Source: CAD feature listing. Evaluate the final solid. Frame: model axes, mm. Face numbers are marked on the shaded views. A direction names the side the tool comes from. Give positions to 0.01 mm unless a question says otherwise; leave off trailing zeros. Order: outer loops, then holes, each group sorted by start corner. A loop starts at its lowest first (then second) coordinate and runs counter-clockwise, first axis right, second up. Notation, with made-up numbers: M -2.75,-4.75 L 12.25,-4.75 A19 ccw 12.25,13.25 Z; hole C 73.5,84.5 d9. An arc over 180 degrees is marked long. Use CSV: the item, a comma, the result in double quotes. Start each with the question number.
Item 1: Section query B-B on y = 0. Return loops of the section in (x, z), and give its area (3 significant figures).
Item 2: Section query C-C on z = -7. Return loops of the section in (x, y).
Item 3: First-contact query: pin 1 (7 mm diameter, centred on x = -3.5, y = -6.5, fed in from +Z); pin 2 (2 mm diameter, centred on x = 1.5, z = -11.5, fed in from -Y); pin 3 (8 mm diameter, centred on y = 6.5, z = 6.5, fed in from -X); pin 4 (5 mm diameter, centred on y = 7.5, z = -10.5, fed in from +X). Flat tips, straight axial feed; report the tip coordinate or a pass-through.
Item 4: Access query for the marked faces 4 and 5. Directions: +Z, -Z, +X, -X, +Y, -Y. A direction counts if a zero-diameter tool reaches every point of the face in a straight line with its end or side. Return the directions, or none.
Item 5: Pull-direction query (Z, two-part tool) for the marked faces 1, 2 and 3; classes: +Z half, -Z half, draft (parallel to the pull), parting line (faces both ways), or undercut.
Item 6: Section query A-A on y = -7.75. Return loops of the section in (x, z), and give its area (3 significant figures).
Item 7: Ray query, probe 1 along Y at (x, z) = (-9.5, -2); probe 2 along Z at (x, y) = (-4.5, 9); probe 3 along X at (y, z) = (-12.5, -6.5). Return the intervals inside material, ascending. Write a range as from..to.
Item 8: Section query D-D on x = 5. Return loops of the section in (y, z).
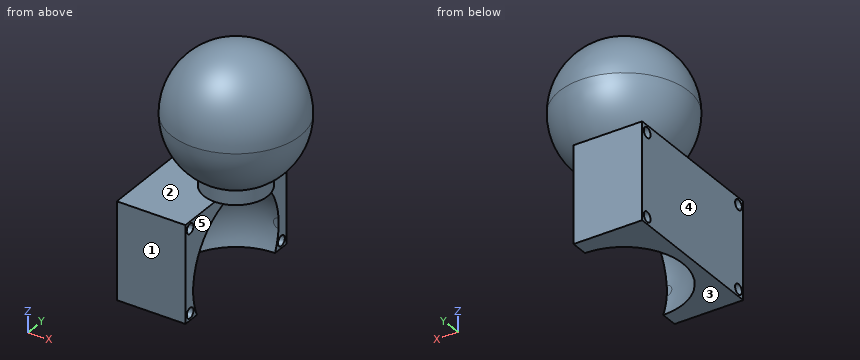
from build123d import *

# Parameters (mm, degrees)
F2_R     = 6.2596868845
F3_DEPTH = 3.048
F4_R     = 1
F5_DEPTH = 13.5


with BuildPart() as f1:
    # F0 (on Right) → F1 (revolve)
    with BuildSketch(Plane.YZ):
        with BuildLine():
            ThreePointArc((0, 1.1509964916), (8.9802561211, 4.8707403706), (12.7, 13.8509964916))
            ThreePointArc((12.7, 13.8509964916), (8.9802561211, 22.8312526127), (0, 26.5509964916))
            Line((0, 26.5509964916), (0, 1.1509964916))
        make_face()
    revolve(axis=Axis((0, 0, 13.8509964916), (0, 0, -1)))

    # F2 (on Top) → F3 (join)
    with BuildSketch(Plane.XY):
        Circle(F2_R)
    extrude(amount=F3_DEPTH)

    # F4 (on Right) → F5 (join)
    with BuildSketch(Plane.YZ):
        with BuildLine():
            Line((-13.603, 0), (-15, 0))
            Line((-15, 0), (-15, -1.397))
            Line((-15, -1.397), (-14.603, -1.397))
            ThreePointArc((-14.603, -1.397), (-14.3101067812, -0.6898932188), (-13.603, -0.397))
            Line((-13.603, -0.397), (-13.603, 0))
        make_face()
        with BuildLine():
            Line((15, 0), (-13.603, 0))
            Line((-13.603, 0), (-13.603, -0.397))
            ThreePointArc((-13.603, -0.397), (-12.8958932188, -0.6898932188), (-12.603, -1.397))
            ThreePointArc((-12.603, -1.397), (-13.603, -2.397), (-14.603, -1.397))
            Line((-14.603, -1.397), (-15, -1.397))
            Line((-15, -1.397), (-15, -12.8640756011))
            Line((-15, -12.8640756011), (-12.6600748075, -12.8640756011))
            ThreePointArc((-12.6600748075, -12.8640756011), (0, -1.170309107), (12.6600748075, -12.8640756011))
            Line((12.6600748075, -12.8640756011), (15, -12.8640756011))
            Line((15, -12.8640756011), (15, 0))
        make_face()
        with Locations((13.5173769371, -1.397)):
            Circle(F4_R, mode=Mode.SUBTRACT)
        with BuildLine():
            Line((-12.6600748075, -12.8640756011), (-15, -12.8640756011))
            Line((-15, -12.8640756011), (-15, -19.05))
            Line((-15, -19.05), (-11.5957234467, -19.05))
            ThreePointArc((-11.5957234467, -19.05), (-12.4208632505, -16.518356711), (-12.7, -13.870309107))
            ThreePointArc((-12.7, -13.870309107), (-12.6900147765, -13.3667964733), (-12.6600748075, -12.8640756011))
        make_face()
        with Locations((-13.603, -17.6556983136)):
            Circle(F4_R, mode=Mode.SUBTRACT)
        with BuildLine():
            Line((15, -19.05), (15, -12.8640756011))
            Line((15, -12.8640756011), (12.6600748075, -12.8640756011))
            ThreePointArc((12.6600748075, -12.8640756011), (12.6900147765, -13.3667964733), (12.7, -13.870309107))
            ThreePointArc((12.7, -13.870309107), (12.4208632505, -16.518356711), (11.5957234467, -19.05))
            Line((11.5957234467, -19.05), (15, -19.05))
        make_face()
        with Locations((13.5173769371, -17.6556983136)):
            Circle(F4_R, mode=Mode.SUBTRACT)
        with BuildLine():
            ThreePointArc((-12.7, -13.870309107), (-12.4208632505, -16.518356711), (-11.5957234467, -19.05))
            Line((-11.5957234467, -19.05), (0, -19.05))
            Line((0, -19.05), (0, -13.870309107))
            Line((0, -13.870309107), (-12.7, -13.870309107))
        make_face()
        with BuildLine():
            Line((0, -19.05), (11.5957234467, -19.05))
            ThreePointArc((11.5957234467, -19.05), (12.4208632505, -16.518356711), (12.7, -13.870309107))
            Line((12.7, -13.870309107), (0, -13.870309107))
            Line((0, -13.870309107), (0, -19.05))
        make_face()
        with BuildLine():
            ThreePointArc((12.6600748075, -12.8640756011), (0, -1.170309107), (-12.6600748075, -12.8640756011))
            ThreePointArc((-12.6600748075, -12.8640756011), (-12.6900147765, -13.3667964733), (-12.7, -13.870309107))
            Line((-12.7, -13.870309107), (0, -13.870309107))
            Line((0, -13.870309107), (12.7, -13.870309107))
            ThreePointArc((12.7, -13.870309107), (12.6900147765, -13.3667964733), (12.6600748075, -12.8640756011))
        make_face()
    extrude(amount=-F5_DEPTH)

    # F4 (on Right) → F6 (revolve, cut)
    with BuildSketch(Plane.YZ):
        with BuildLine():
            ThreePointArc((12.6600748075, -12.8640756011), (0, -1.170309107), (-12.6600748075, -12.8640756011))
            ThreePointArc((-12.6600748075, -12.8640756011), (-12.6900147765, -13.3667964733), (-12.7, -13.870309107))
            Line((-12.7, -13.870309107), (0, -13.870309107))
            Line((0, -13.870309107), (12.7, -13.870309107))
            ThreePointArc((12.7, -13.870309107), (12.6900147765, -13.3667964733), (12.6600748075, -12.8640756011))
        make_face()
    revolve(axis=Axis((0, 0, -13.870309107), (0, 1, 0)), mode=Mode.SUBTRACT)


solid = f1.part
Verdict:
1,outline,"M -13.5,-19.05 L -11.6,-19.05 A12.7 cw 0,-1.17 L 0,0 L 6.26,0 L 6.26,2.8 A12.7 ccw long -6.26,2.8 L -6.26,0 L -13.5,0 Z"
1,area,"594 mm2"
2,outline,"M -13.5,-15 L 0,-15 L 0,-10.68 A10.68 cw 0,10.68 L 0,15 L -13.5,15 Z"
3,pin 1,"z = 25.94"
3,pin 2,"through"
3,pin 3,"x = -11.29"
3,pin 4,"x = -6.81"
4,face 4,"+Z, -Z, -X, +Y, -Y"
4,face 5,"-Z, +X, +Y, -Y"
5,face 1,"draft"
5,face 2,"undercut"
5,face 3,"-Z half"
6,outline,"M -13.5,-19.05 L -8.63,-19.05 A10.06 cw 0,-3.81 L 0,0 L -13.5,0 Z; C 0,13.85 d20.12"
6,area,"446 mm2"
7,probe 1,"-15..-14.4, -12.81..12.72, 14.32..15"
7,probe 2,"-6.12..0, 6.1..21.6"
7,probe 3,"-13.5..0"
8,outline,"M -3.77,0 L 3.77,0 L 3.77,2.8 A11.67 ccw long -3.77,2.8 Z"
